Read the model definition and answer for the solid it produces. Units are mm, in the model's axes. A direction names the side the tool comes from. Give positions to 0.01 mm unless a question says otherwise; leave off trailing zeros. Write each loop counter-clockwise with the first axis right and the second up, starting at its lowest first coordinate (ties: lowest second). Pieces come first, ordered by that corner, then holes. Notation, with made-up numbers: (47, 59.5) - (64, 59.5) arc R24 ccw to (64, 71.5) - close; hole circle Ø9 at (-37.75, 84.25). An arc over 180 degrees is marked (long way). Answer as a JSON object with one key per item and string values. Group by question number.
Autodesk Inventor part; units mm, degrees
ref_plane "YZ Plane" through (0, 0, 0) normal (1, 0, 0) x (0, 1, 0)
ref_plane "XZ Plane" through (0, 0, 0) normal (0, 1, 0) x (-1, 0, 0)
ref_plane "XY Plane" through (0, 0, 0) normal (0, 0, 1) x (1, 0, 0)
ref_plane "Work Plane1" through (0, 0, 1) normal (0, 0, 1) x (1, 0, 0)
sketch "Sketch2" plane through (0, 0, 1) normal (0, 0, 1) x (1, 0, 0)
  circle A0 centre (-25.527, 21.082) radius 1.5875
  circle A1 centre (-25.527, -29.718) radius 1.5875
  circle A2 centre (21.463, 21.082) radius 1.5875
  circle A3 centre (21.463, -29.718) radius 1.5875
  circle A4 centre (20.213, 14.652) radius 0.595
  circle A5 centre (20.213, 9.652) radius 0.595
  circle A6 centre (20.213, 4.652) radius 0.595
  circle A7 centre (-25.527, 4.572) radius 0.51
  circle A8 centre (-25.527, 2.032) radius 0.51
  circle A9 centre (-25.527, -0.508) radius 0.51
  circle A10 centre (-25.527, -9.398) radius 0.51
  circle A11 centre (-25.527, -6.858) radius 0.51
  circle A12 centre (7.493, 13.462) radius 0.5
  circle A13 centre (10.033, 13.462) radius 0.5
  circle A14 centre (12.573, 13.462) radius 0.5
  circle A15 centre (12.773, -3.988) radius 0.5
  circle A16 centre (7.693, -1.448) radius 0.5
  circle A17 centre (16.273, -30.798) radius 0.5
  circle A18 centre (13.733, -30.798) radius 0.5
  circle A19 centre (4.273, -30.798) radius 0.5
  circle A20 centre (1.733, -30.798) radius 0.5
  circle A21 centre (7.693, -3.988) radius 0.5
  circle A22 centre (5.153, -1.448) radius 0.5
  circle A23 centre (5.153, -3.988) radius 0.5
  circle A24 centre (12.773, -1.448) radius 0.5
  circle A25 centre (10.233, -3.988) radius 0.5
  circle A26 centre (10.233, -1.448) radius 0.5
  circle A27 centre (-19.427, 6.092) radius 0.5
  circle A28 centre (-19.427, 3.552) radius 0.5
  circle A29 centre (-19.427, 1.012) radius 0.5
  circle A30 centre (-19.427, -1.528) radius 0.5
  circle A31 centre (-19.427, -4.068) radius 0.5
  circle A32 centre (-19.427, -6.608) radius 0.5
  circle A33 centre (-19.427, -9.148) radius 0.5
  circle A34 centre (-19.427, -11.688) radius 0.5
  circle A35 centre (-19.427, -14.228) radius 0.5
  circle A36 centre (-19.427, -16.768) radius 0.5
  circle A37 centre (-19.427, -19.308) radius 0.5
  circle A38 centre (-19.427, -21.848) radius 0.5
  circle A39 centre (-19.427, -24.388) radius 0.5
  circle A40 centre (-19.427, -26.928) radius 0.5
  circle A41 centre (-19.427, -29.468) radius 0.5
  circle A42 centre (-4.187, 6.092) radius 0.5
  circle A43 centre (-4.187, 3.552) radius 0.5
  circle A44 centre (-4.187, 1.012) radius 0.5
  circle A45 centre (-4.187, -1.528) radius 0.5
  circle A46 centre (-4.187, -4.068) radius 0.5
  circle A47 centre (-4.187, -6.608) radius 0.5
  circle A48 centre (-4.187, -9.148) radius 0.5
  circle A49 centre (-4.187, -11.688) radius 0.5
  circle A50 centre (-4.187, -14.228) radius 0.5
  circle A51 centre (-4.187, -16.768) radius 0.5
  circle A52 centre (-4.187, -19.308) radius 0.5
  circle A53 centre (-4.187, -21.848) radius 0.5
  circle A54 centre (-4.187, -24.388) radius 0.5
  circle A55 centre (-4.187, -26.928) radius 0.5
  circle A56 centre (-4.187, -29.468) radius 0.5
  circle A57 centre (0.893, 13.462) radius 0.405
  circle A58 centre (3.433, 13.462) radius 0.405
  circle A59 centre (1.143, 5.842) radius 0.405
  circle A60 centre (3.683, 5.842) radius 0.405
  circle A61 centre (9.143, 21.672) radius 0.4
  circle A62 centre (10.413, 19.732) radius 0.4
  circle A63 centre (11.933, 21.672) radius 0.4
  circle A64 centre (13.463, 19.732) radius 0.4
  circle A65 centre (-24.257, -23.368) radius 0.375
  circle A66 centre (-24.257, -20.828) radius 0.375
  circle A67 centre (-24.257, -18.288) radius 0.375
  circle A68 centre (-25.527, 9.942) radius 0.35
  circle A69 centre (-25.527, 11.442) radius 0.35
  circle A70 centre (-25.527, 12.942) radius 0.35
  circle A71 centre (-25.527, 14.442) radius 0.35
  circle A72 centre (-16.002, 5.842) radius 0.254
  circle A73 centre (-3.302, 7.747) radius 0.254
  circle A74 centre (-12.192, 4.572) radius 0.254
  circle A75 centre (-5.842, -1.778) radius 0.254
  circle A76 centre (-12.192, -3.683) radius 0.254
  circle A77 centre (-19.812, 9.017) radius 0.254
  circle A78 centre (-22.352, -11.303) radius 0.254
  circle A79 centre (-21.717, -7.493) radius 0.254
  circle A80 centre (-10.922, -12.573) radius 0.254
  circle A81 centre (-10.922, 7.112) radius 0.254
  circle A82 centre (-9.652, -11.303) radius 0.254
  circle A83 centre (-7.112, 9.017) radius 0.254
  line L0 (25.273, 24.892) -> (-29.337, 24.892)
  line L1 (-29.337, 24.892) -> (-29.337, -33.528)
  line L2 (-29.337, -33.528) -> (25.273, -33.528)
  line L3 (25.273, -33.528) -> (25.273, 24.892)
  line L4 (18, -43) -> (18, 0.1016)
  line L5 (-0.1016, 0.1016) -> (-0.1016, -43)
  line L6 (18, 0.1016) -> (-0.1016, 0.1016)
  line L7 (-0.1016, 0.1016) -> (-0.1016, -33.3629)
  line L8 (-0.1016, -33.3629) -> (18, -33.3629)
  line L9 (18, -33.3629) -> (18, 0.1016)
  point P0 (0, 0)
  dimension "d3" = 33.4645
extrude "Extrusion2" add sketch "Sketch2" along normal blind 1.3716 contours L8 L5 L6 L4
sketch "Sketch3" plane through (0, 0, 2.3716) normal (0, 0, 1) x (1, 0, 0)
  circle A0 centre (10.233, -1.448) radius 0.5
  circle A1 centre (10.233, -3.988) radius 0.5
  circle A2 centre (12.773, -1.448) radius 0.5
  circle A3 centre (5.153, -3.988) radius 0.5
  circle A4 centre (5.153, -1.448) radius 0.5
  circle A5 centre (7.693, -3.988) radius 0.5
  circle A6 centre (1.733, -30.798) radius 0.5
  circle A7 centre (4.273, -30.798) radius 0.5
  circle A8 centre (13.733, -30.798) radius 0.5
  circle A9 centre (16.273, -30.798) radius 0.5
  circle A10 centre (7.693, -1.448) radius 0.5
  circle A11 centre (12.773, -3.988) radius 0.5
  line L0 (18, 0.1016) -> (-0.1016, 0.1016)
  line L1 (-0.1016, 0.1016) -> (-0.1016, -33.3629)
  line L2 (-0.1016, -33.3629) -> (18, -33.3629)
  line L3 (18, -33.3629) -> (18, 0.1016)
  line L4 (16.476, -28.0924) -> (1.4265, -28.0924)
  line L5 (1.4265, -28.0924) -> (1.4265, -6.0198)
  line L6 (1.4265, -6.0198) -> (16.476, -6.0198)
  line L7 (16.476, -6.0198) -> (16.476, -28.0924)
  point P0 (0, 0)
  dimension "d6" = 15.0495
  dimension "d7" = 22.0726
  dimension "d8" = 5.2705
  dimension "d9" = 1.524
extrude "Extrusion3" add sketch "Sketch3" along normal blind 2.6543 contours L4 L5 L6 L7
fillet "Fillet1" radius 0.2286 8 edges at (16.476, -17.0561, 5.0259) (8.9513, -6.0198, 5.0259) (1.4265, -17.0561, 5.0259) (8.9513, -28.0924, 5.0259) (16.476, -28.0924, 3.6988) (1.4265, -28.0924, 3.6988) (16.476, -6.0198, 3.6988) (1.4265, -6.0198, 3.6988)
sketch "Sketch4" plane through (0, 0, 5.0259) normal (0, 0, 1) x (1, 0, 0)
  line L0 (16.2703, -6.3451) -> (16.2703, -27.5869) construction
  line L1 (16.2703, -27.5869) -> (1.6519, -27.5869) construction
  line L2 (1.6519, -27.5869) -> (1.6519, -6.3451) construction
  line L3 (1.6519, -6.3451) -> (16.2703, -6.3451) construction
  point P0 (0, 0)
decal "Decal1"
properties part number "E01-ML01DP5"
1) Find section D-D, the plane x = 10.25. Write down the section's boundary in (y, z), and give its area (3 significant figures).
2) Find section B-B, the plane x = 3. Write down the section's boundary in (y, z).
3) Which of the six approach directions +Z, -Z, +X, -X, +Y, -Y give full straight-line access (tool end or side, diameter ignored) to faces 4 (the flat face through (16.476, -17, 4)), 5 (the flat face through (9, -6.02, 4)), 6 (the flat face through (17, -16, 2.372))?
4) Flat-ended cylindrical pins translate along their axes: pin 1 Ø0.7 at (y, z) = (-21.5, 3.5) entering from -X; pin 2 Ø10 at (x, y) = (9.5, -29) entering from +Z; pin 3 Ø1.2 at (x, z) = (12.5, 4) entering from +Y; pin 4 Ø0.7 at (x, z) = (8, 3.5) entering from -Y. Find the tip coordinate at first contact, or state that the pin passes through.
5) Find the intervals of material crossed by line 1 (Y direction, x = 10.5, z = 1.2); line 2 (X direction, y = -26.5, z = 3.9); line 3 (Y direction, x = 8.5, z = 3.65), in increasing order. Write a range as [from, to].
6) For a pull along Y with two mould halves and no side action, classify faces 1 (the cylindrical face through (7.193, -1.47, 1.676)), 2 (the flat face through (9, -16, 1)), 3 (the flat face through (9, -33.363, 2)) as released by +Y, released by -Y, zero draft, split by the parting line, or undercut.
7) Find section C-C, the plane y = -17. Write down the section's boundary in (x, z).
8) Find section A-A, the plane z = 4. Write down the section's boundary in (x, y).
Values follow:
{
 "1": {"outline": "(-33.36, 1) - (-4.49, 1) - (-4.49, 2.37) - (-6.02, 2.37) - (-6.02, 4.8) arc R0.23 ccw to (-6.25, 5.03) - (-27.86, 5.03) arc R0.23 ccw to (-28.09, 4.8) - (-28.09, 2.37) - (-33.36, 2.37) - close; (-3.49, 1) - (-1.95, 1) - (-1.95, 2.37) - (-3.49, 2.37) - close; (-0.95, 1) - (0.1, 1) - (0.1, 2.37) - (-0.95, 2.37) - close", "area": "102 mm2"},
 "2": {"outline": "(-33.36, 1) - (0.1, 1) - (0.1, 2.37) - (-6.02, 2.37) - (-6.02, 4.8) arc R0.23 ccw to (-6.25, 5.03) - (-27.86, 5.03) arc R0.23 ccw to (-28.09, 4.8) - (-28.09, 2.37) - (-33.36, 2.37) - close"},
 "3": {"face 4": "+Z, +X, +Y, -Y", "face 5": "+Z, +X, -X, +Y", "face 6": "+Z"},
 "4": {"pin 1": "stops at x = 1.43", "pin 2": "stops at z = 5.03", "pin 3": "stops at y = -6.02", "pin 4": "stops at y = -28.09"},
 "5": {"line 1": "y = [-33.36, -4.41], [-3.57, -1.87], [-1.03, 0.1]", "line 2": "x = [1.43, 16.48]", "line 3": "y = [-28.09, -6.02]"},
 "6": {"face 1": "undercut", "face 2": "zero draft", "face 3": "released by -Y"},
 "7": {"outline": "(-0.1, 1) - (18, 1) - (18, 2.37) - (16.48, 2.37) - (16.48, 4.8) arc R0.23 ccw to (16.25, 5.03) - (1.66, 5.03) arc R0.23 ccw to (1.43, 4.8) - (1.43, 2.37) - (-0.1, 2.37) - close"},
 "8": {"outline": "(1.43, -27.86) arc R0.23 ccw to (1.66, -28.09) - (16.25, -28.09) arc R0.23 ccw to (16.48, -27.86) - (16.48, -6.25) arc R0.23 ccw to (16.25, -6.02) - (1.66, -6.02) arc R0.23 ccw to (1.43, -6.25) - close"}
}
